from build123d import *

# Parameters (mm, degrees)
F1_DEPTH = 19.05
F3_R     = 3.175
F4_DEPTH = 19.051
F6_DEPTH = 19.051


with BuildPart() as f1:
    # F0 (on Top) → F1 (new body)
    with BuildSketch(Plane.XY):
        with BuildLine():
            ThreePointArc((38.975515, -3.440669), (40.835387, 1.049459), (45.325515, 2.909331))
            Line((45.325515, 2.909331), (61.458508, 2.909331))
            ThreePointArc((61.458508, 2.909331), (67.341307, 6.868686), (65.888014, 13.809274))
            Line((65.888014, 13.809274), (2.81784, 75.209965))
            ThreePointArc((2.81784, 75.209965), (-1.696828, 77.009451), (-6.161608, 75.089527))
            Line((-6.161608, 75.089527), (-65.937009, 13.688836))
            ThreePointArc((-65.937009, 13.688836), (-67.237273, 6.790005), (-61.387065, 2.909331))
            Line((-61.387065, 2.909331), (-44.756616, 2.909331))
            ThreePointArc((-44.756616, 2.909331), (-40.285175, 1.068068), (-38.406835, -3.387924))
            Line((-38.406835, -3.387924), (-38.091605, -41.337081))
            ThreePointArc((-38.091605, -41.337081), (-36.213265, -45.793073), (-31.741824, -47.634335))
            Line((-31.741824, -47.634335), (32.625515, -47.634335))
            ThreePointArc((32.625515, -47.634335), (37.115643, -45.774463), (38.975515, -41.284335))
            Line((38.975515, -41.284335), (38.975515, -3.440669))
        make_face()
    extrude(amount=F1_DEPTH)

    # F3 (on face) → F4 (cut, through all)
    with BuildSketch(Plane.XY.offset(19.05)):
        with Locations((-56.677773, 11.351841)):
            Circle(F3_R)
        with Locations((30.4104, -39.055706)):
            Circle(F3_R)
    extrude(amount=-F4_DEPTH, mode=Mode.SUBTRACT)

    # F5 (on face) → F6 (cut, through all)
    with BuildSketch(Plane.XY.offset(19.05)):
        with BuildLine():
            Line((-8.287639, 65.80173), (-47.495655, 22.642287))
            ThreePointArc((-47.495655, 22.642287), (-48.781233, 16.252613), (-43.760738, 12.096261))
            Line((-43.760738, 12.096261), (-31.995475, 10.286895))
            Line((-31.995475, 10.286895), (-31.995475, -26.759769))
            ThreePointArc((-31.995475, -26.759769), (-30.135603, -31.249897), (-25.645475, -33.109769))
            Line((-25.645475, -33.109769), (24.530177, -33.109769))
            ThreePointArc((24.530177, -33.109769), (29.020305, -31.249897), (30.880177, -26.759769))
            Line((30.880177, -26.759769), (30.880177, 11.435365))
            Line((30.880177, 11.435365), (39.708046, 11.435365))
            ThreePointArc((39.708046, 11.435365), (45.568366, 15.340135), (44.221378, 22.252168))
            Line((44.221378, 22.252168), (0.925822, 65.998721))
            ThreePointArc((0.925822, 65.998721), (-3.723247, 67.880467), (-8.287639, 65.80173))
        make_face()
    extrude(amount=-F6_DEPTH, mode=Mode.SUBTRACT)


solid = f1.part
Build history of the part. All positions in model axes, mm. A direction names the side the tool comes from. Round coordinates to 2 decimals unless told otherwise and drop trailing zeros. Write each loop counter-clockwise with the first axis right and the second up, starting at its lowest first coordinate (ties: lowest second). Pieces come first, ordered by that corner, then holes. Notation, with made-up numbers: M 55.5,72 L 83.5,72 A25 cw 83.5,110 Z; hole C 63,-2.5 d11. An arc over 180 degrees is marked long. Answer as a JSON object with one key per item and string values. Group by question number.
(1) Which spindle directions (+Z, -Z, +X, -X, +Y, -Y) get a long thin tool onto all of the face, cutting with end or side? Do faces 5 (the cylindrical face through (-2, 77, 9)), 6 (the flat face through (-53, 2.909, 9)), 7 (the cylindrical face through (45.527, 15.244, 9.658)). Say none if no direction does.
(2) Flat gauge pins, fed straight in: pin 1 (6 mm diameter, centred on x = -48.5, z = 4.5, fed in from +Y); pin 2 (3 mm diameter, centred on y = 3.5, z = 14.5, fed in from -X); pin 3 (3 mm diameter, centred on y = 8.5, z = 11.5, fed in from +X); pin 4 (9.5 mm diameter, centred on y = -4.5, z = 12, fed in from +X). Where does each tip first touch, or does it go through?
(3) Cut at D-D (x = 53). Give the cut face in (y, z).
(4) Drill centre lines: L1, parallel to Y at x = 32, z = 7.5; L2, parallel to X at y = -6, z = 11.25; L3, parallel to Y at x = 31, z = 18. Where is each one in solid material? Low to high.
(5) Cut at A-A (x = -22). Give the cut face in (y, z), and give its area (3 significant figures).
(6) Cut at B-B (y = 58). Give the cut face in (x, z), and give its area (3 significant figures).
(7) Cut at C-C (z = 13.25). Give the number of separate pieces and of enclosed holes in the cut face, and give its area (3 significant figures).
(8) Mould opens along Y. For faces 1 (the flat face through (38.976, -23, 9)), 2 (the cylindrical face through (28.97, -31.3, 9.66)), 3 (the flat face through (53, 2.909, 9)), 4 (the cylindrical face through (-67.28, 6.89, 9.39)) say: pulls with the +Y half, pulls with the -Y half, needs draft (parallel to the pull), parting line crosses it, or undercut.
Responses:
{
 "1": {"face 5": "+Z, -Z, +Y", "face 6": "+Z, -Z, -X, -Y", "face 7": "+Z, -Z"},
 "2": {"pin 1": "stops at y = 34.68", "pin 2": "stops at x = -66.1", "pin 3": "stops at x = 67.81", "pin 4": "stops at x = 40.16"},
 "3": {"outline": "M 2.91,0 L 26.36,0 L 26.36,19.05 L 2.91,19.05 Z"},
 "4": {"L1": "y = -47.63 to -41.8, -36.31 to 11.44, 34.6 to 46.8", "L2": "x = -38.39 to -32, 30.88 to 38.98", "L3": "y = -47.63 to -42.18, -35.94 to 11.44, 35.61 to 47.77"},
 "5": {"outline": "M -47.63,0 L -33.11,0 L -33.11,19.05 L -47.63,19.05 Z; M 50.71,0 L 58.82,0 L 58.82,19.05 L 50.71,19.05 Z", "area": "431 mm2"},
 "6": {"outline": "M -22.8,0 L -15.38,0 L -15.38,19.05 L -22.8,19.05 Z; M 8.84,0 L 20.5,0 L 20.5,19.05 L 8.84,19.05 Z", "area": "363 mm2"},
 "7": {"separate pieces": "1", "enclosed holes": "3", "area": "3,610 mm2"},
 "8": {"face 1": "needs draft", "face 2": "undercut", "face 3": "pulls with the -Y half", "face 4": "parting line crosses it"}
}
